Part print with two shaded views. Sizes in mm from the minimum x, y, z corner. Give positions to 0.01 mm unless a question says otherwise; leave off trailing zeros. Order: outer loops, then holes, each group sorted by start corner. A loop starts at its lowest first (then second) coordinate and runs counter-clockwise, first axis right, second up. Notation, with made-up numbers: M -6,-24.5 L 17,-24.5 A14 ccw 17,0.5 Z; hole C -33.5,-39.5 d10. An arc over 180 degrees is marked long. Answer as CSV lines item,"result".
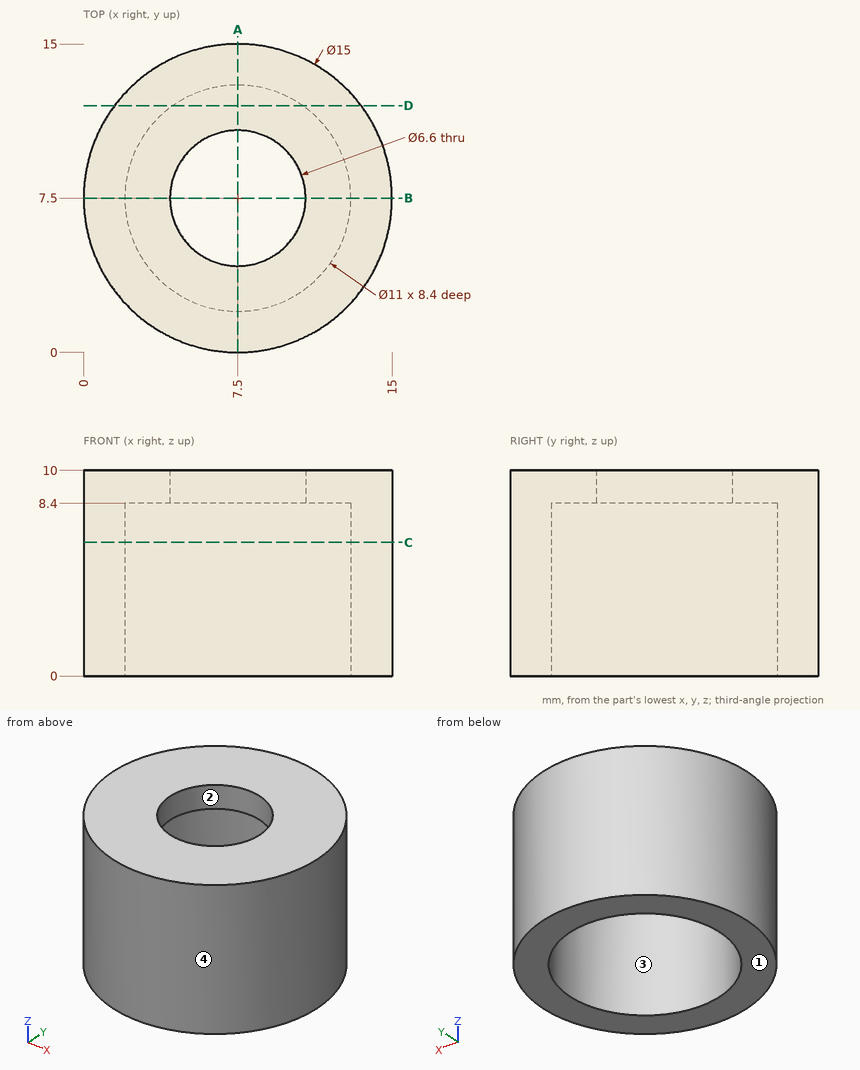
Item 1: Drop flat-ended pins along their axis: pin 1 (3 mm diameter, centred on x = 13.5, z = 8, fed in from +Y); pin 2 (1 mm diameter, centred on y = 4.5, z = 4, fed in from +X); pin 3 (1.5 mm diameter, centred on y = 4.5, z = 5, fed in from -X); pin 4 (8 mm diameter, centred on x = 4, y = 10, fed in from -Z). Give the stop position or say it passes through.
Geometry says:
pin 1,"stops at y = 13.5"
pin 2,"stops at x = 14.57"
pin 3,"stops at x = 0.35"
pin 4,"stops at z = 0"
Item 2: Band-saw the part on A-A (x = 7.5). Give the cut face in (y, z).
Geometry says:
outline,"M 0,0 L 2,0 L 2,8.4 L 4.2,8.4 L 4.2,10 L 0,10 Z; M 10.8,8.4 L 13,8.4 L 13,0 L 15,0 L 15,10 L 10.8,10 Z"
Item 3: Band-saw the part on C-C (z = 6.5). Give the cut face in (x, y).
Geometry says:
outline,"C 7.5,7.5 d15; hole C 7.5,7.5 d11"
Item 4: Probe line 1 along Y through (x, z) = (7.5, 6); line 2 along Y through (x, z) = (7.5, 9.65); line 3 along Z through (x, y) = (6.25, 4). List the from-to ranges inside material, lowest first. Write a range as from..to.
Geometry says:
line 1,"y = 0..2, 13..15"
line 2,"y = 0..4.2, 10.8..15"
line 3,"z = 8.4..10"
Item 5: Band-saw the part on D-D (y = 12). Give the cut face in (x, z).
Geometry says:
outline,"M 1.5,0 L 4.34,0 L 4.34,8.4 L 10.66,8.4 L 10.66,0 L 13.5,0 L 13.5,10 L 1.5,10 Z"
Item 6: Pull direction Y, two halves, no side cores. Call the marked faces 1, 2, 3 and 4: released by +Y, released by -Y, zero draft, split by the parting line, or undercut.
Geometry says:
face 1,"zero draft"
face 2,"undercut"
face 3,"undercut"
face 4,"split by the parting line"
